The model under review builds one solid part; all positions refer to its coordinate system, in mm. A direction names the side the tool comes from. Round coordinates to 2 decimals unless told otherwise and drop trailing zeros. Write each loop counter-clockwise with the first axis right and the second up, starting at its lowest first coordinate (ties: lowest second). Pieces come first, ordered by that corner, then holes. Notation, with made-up numbers: (-0.5, 35.5) -> (42.5, 35.5) arc R34 ccw to (42.5, 73.5) -> close; hole circle Ø2 at (51.5, -7.5). An arc over 180 degrees is marked (long way). Return JSON: item names as keys, results as strings. Group by question number.
1. Take a section at D-D, the plane x = 16.5. Write out the cut boundary in (y, z).
2. Take a section at B-B, the plane z = -5.2. Give the number of separate pieces and of enclosed holes in the cut face, then the cut area to 3 significant figures.
3. Take a section at A-A, the plane x = 0. Write out the cut boundary in (y, z).
4. Clearance check with flat-ended pins moving along their axes: P1, Ø6.5, axis at x = 2.5, z = 0.5, coming from the +Y side; P2, Ø3, axis at x = 4, z = -7.5, coming from the -Y side; P3, Ø2, axis at y = 3.5, z = 2.5, coming from the -X side; P4, Ø2, axis at x = 16, z = -6.5, coming from the -Y side. State where each tip first meets the part, or that it passes through.
5. Mouldability with a two-part tool opening along X and no side actions: class faces 1 (the flat face through (0, 2, -11.829)), 2 (the cylindrical face through (18.2, 5.479, -2.317)), 3 (the flat face through (-23.442, 2, -1)) as pulls with the +X half, pulls with the -X half, needs draft (parallel to the pull), parting line crosses it, or undercut.
6. Tool access review of faces 4 (the cylindrical face through (-15.443, 1.479, -4.324)), 5 (the flat face through (9, 1, -2.4)), 6 (the cylindrical face through (-18.57, 3.51, -3.59)): name each direction out of +Z, -Z, +X, -X, +Y, -Y from which nothing blocks a thin tool from reaching the whole face with its end or side.
7. Take a section at C-C, the plane y = 4.5. Write out the cut boundary in (x, z).
8. For line 1 along Z through (x, y) = (0, 3.65); line 2 along Z through (x, y) = (12, 2.25); line 3 along X through (y, z) = (2.25, 4.5), list the stretches that pass through material, from the lowest coordinate up. Write a range as from..to.
from build123d import *

# Parameters (mm, degrees)
SKETCH2_W           = 46.883828082
SKETCH2_H           = 21
SKETCH2_R           = 2
SKETCH2_R_2         = 2.054050428
SKETCH2_R_3         = 3.25
BOSS_EXTRUDE2_DEPTH = 4
SKETCH2_2_R         = 3.25
BOSS_EXTRUDE3_DEPTH = 7
CUT_EXTRUDE1_REACH  = 9
SKETCH1_R           = 1.75
HOLE1_D             = 4
HOLE1_DEPTH         = 4
HOLE1_CBORE_D       = 9
HOLE1_CBORE_DEPTH   = 1
FILLET1_R           = 8
SKETCH6_R           = 1.75
CUT_EXTRUDE2_DEPTH  = 2.5


with BuildPart() as part:
    # Sketch2 → Boss-Extrude2 (new body)
    with BuildSketch(Plane(origin=(0, 0, 0), x_dir=(1, 0, 0), z_dir=(0, 1, 0))):
        with Locations((0, 1.329477691)):
            Rectangle(SKETCH2_W, SKETCH2_H)
        with Locations((-14.997509842, -3.670522309)):
            Circle(SKETCH2_R, mode=Mode.SUBTRACT)
        with Locations((-14.997509842, 6.329477691)):
            Circle(SKETCH2_R_2, mode=Mode.SUBTRACT)
        with Locations((-2.8, 5.2)):
            Circle(SKETCH2_R_3, mode=Mode.SUBTRACT)
        with Locations((0, -3.943832634)):
            Circle(SKETCH2_R, mode=Mode.SUBTRACT)
        with Locations((16.7, 5.2)):
            Circle(SKETCH2_R_3, mode=Mode.SUBTRACT)
    extrude(amount=BOSS_EXTRUDE2_DEPTH)

    # Sketch2<2> → Boss-Extrude3 (add)
    with BuildSketch(Plane(origin=(0, 0, 0), x_dir=(1, 0, 0), z_dir=(0, 1, 0))):
        with Locations((-2.8, 5.2)):
            Circle(SKETCH2_2_R)
        with Locations((16.7, 5.2)):
            Circle(SKETCH2_2_R)
    extrude(amount=BOSS_EXTRUDE3_DEPTH)

    # Sketch1 → Cut-Extrude1 (cut, up to next)
    with BuildSketch(Plane(origin=(0, 0, 0), x_dir=(1, 0, 0), z_dir=(0, 1, 0)), mode=Mode.PRIVATE) as cut_extrude1_sk1:
        with Locations((-2.8, 5.2)):
            Circle(SKETCH1_R)
    cut_extrude1_tool1 = extrude(cut_extrude1_sk1.sketch, amount=CUT_EXTRUDE1_REACH, mode=Mode.PRIVATE) & part.part
    add(cut_extrude1_tool1.solids().sort_by_distance((-2.8, 0, -5.2))[0], mode=Mode.SUBTRACT)
    # Sketch1 → Cut-Extrude1 (cut, up to next)
    with BuildSketch(Plane(origin=(0, 0, 0), x_dir=(1, 0, 0), z_dir=(0, 1, 0)), mode=Mode.PRIVATE) as cut_extrude1_sk2:
        with Locations((16.7, 5.2)):
            Circle(SKETCH1_R)
    cut_extrude1_tool2 = extrude(cut_extrude1_sk2.sketch, amount=CUT_EXTRUDE1_REACH, mode=Mode.PRIVATE) & part.part
    add(cut_extrude1_tool2.solids().sort_by_distance((16.7, 0, -5.2))[0], mode=Mode.SUBTRACT)

    # Hole1
    with Locations(Plane(origin=(0, 4, 0), x_dir=(1, 0, 0), z_dir=(0, 1, 0))):
        with Locations((0, -3.943832634), (15, -3.943832634), (-14.997509842, -3.670522309), (-14.997509842, 6.329477691)):
            CounterBoreHole(HOLE1_D / 2, HOLE1_CBORE_D / 2, HOLE1_CBORE_DEPTH, depth=HOLE1_DEPTH)

    # Fillet1
    fillet1_edges = [part.edges().sort_by_distance(p)[0] for p in [
        (23.441914041, 2, -11.829477691),
        (23.441914041, 2, 9.170522309),
        (-23.441914041, 2, 9.170522309),
        (-23.441914041, 2, -11.829477691),
    ]]
    fillet(fillet1_edges, radius=FILLET1_R)

    # Sketch6 → Cut-Extrude2 (cut)
    with BuildSketch(Plane.XZ):
        with BuildLine():
            Line((19.933161507, -5.2), (18.316580754, -8))
            Line((18.316580754, -8), (22.268827229, -8))
            ThreePointArc((22.268827229, -8), (23.143060238, -5.995660336), (23.441914041, -3.829477691))
            Line((23.441914041, -3.829477691), (23.441914041, -2.4))
            Line((23.441914041, -2.4), (18.316580754, -2.4))
            Line((18.316580754, -2.4), (19.933161507, -5.2))
        make_face()
        Polygon((13.466838493, -5.2), (15.083419246, -8), (18.316580754, -8), (19.933161507, -5.2), (18.316580754, -2.4), (15.083419246, -2.4), align=None)
        with Locations((16.7, -5.2)):
            Circle(SKETCH6_R, mode=Mode.SUBTRACT)
        Polygon((0.433161507, -5.2), (-1.183419246, -8), (15.083419246, -8), (13.466838493, -5.2), (15.083419246, -2.4), (-1.183419246, -2.4), align=None)
        Polygon((-4.416580754, -2.4), (-6.033161507, -5.2), (-4.416580754, -8), (-1.183419246, -8), (0.433161507, -5.2), (-1.183419246, -2.4), align=None)
        with Locations((-2.8, -5.2)):
            Circle(SKETCH6_R, mode=Mode.SUBTRACT)
        Polygon((-6.033161507, -2.4), (-6.033161507, -5.2), (-4.416580754, -2.4), align=None)
        Polygon((-6.033161507, -5.2), (-6.033161507, -8), (-4.416580754, -8), align=None)
    extrude(amount=-CUT_EXTRUDE2_DEPTH, mode=Mode.SUBTRACT)


solid = part.part
Output:
{
 "1": {"outline": "(0, -11.76) -> (4, -11.76) -> (4, -8.44) -> (7, -8.44) -> (7, -6.94) -> (2.5, -6.94) -> (2.5, -8) -> (0, -8) -> close; (0, -2.4) -> (2.5, -2.4) -> (2.5, -3.46) -> (7, -3.46) -> (7, -1.96) -> (4, -1.96) -> (4, -0.3) -> (3, -0.3) -> (3, 2.62) -> (0, 2.62) -> close; (0, 5.27) -> (3, 5.27) -> (3, 8.19) -> (4, 8.19) -> (4, 9.1) -> (0, 9.1) -> close"},
 "2": {"separate pieces": "4", "enclosed holes": "0", "area": "102 mm^2"},
 "3": {"outline": "(0, -11.83) -> (4, -11.83) -> (4, -6.85) -> (7, -6.85) -> (7, -3.55) -> (4, -3.55) -> (4, -0.56) -> (3, -0.56) -> (3, 1.94) -> (0, 1.94) -> (0, -2.4) -> (2.5, -2.4) -> (2.5, -8) -> (0, -8) -> close; (0, 5.94) -> (3, 5.94) -> (3, 8.44) -> (4, 8.44) -> (4, 9.17) -> (0, 9.17) -> close"},
 "4": {"P1": "stops at y = 4", "P2": "stops at y = 0", "P3": "stops at x = -23.44", "P4": "stops at y = 2.5"},
 "5": {"face 1": "needs draft", "face 2": "undercut", "face 3": "pulls with the -X half"},
 "6": {"face 4": "+Y, -Y", "face 5": "+X, -Y", "face 6": "+Y"},
 "7": {"outline": "circle Ø6.5 at (-2.8, -5.2); circle Ø6.5 at (16.7, -5.2); hole circle Ø3.5 at (-2.8, -5.2); hole circle Ø3.5 at (16.7, -5.2)"},
 "8": {"line 1": "z = -11.83..-0.56, 8.44..9.17", "line 2": "z = -11.83..-8, -2.4..9.17", "line 3": "x = -22.72..-16.82, -13.18..-1.92, 1.92..13.08, 16.92..22.72"}
}
